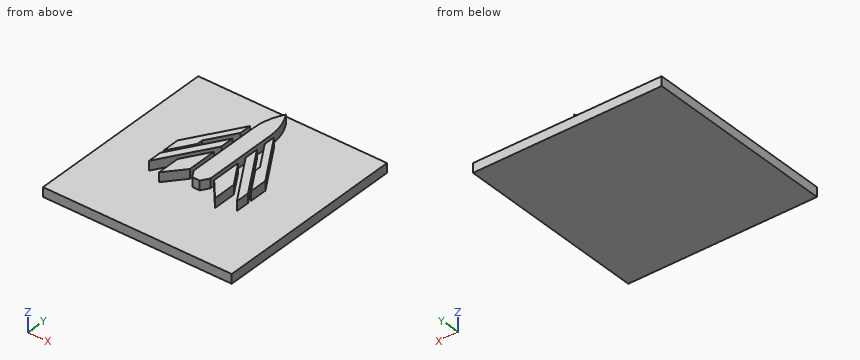
```python
from build123d import *

# Parameters (mm, degrees)
PAD_DEPTH    = 10
SKETCH002_W  = 201.991504
SKETCH002_H  = 207.023942
PAD001_DEPTH = 10
PAD002_DEPTH = 10
PAD003_DEPTH = 10
PAD004_DEPTH = 10


with BuildPart() as part:
    # Sketch → Pad (new body)
    with BuildSketch(Plane.XY):
        with BuildLine():
            Line((-9, 62.657148), (-9, -17.342852))
            Line((-9, -17.342852), (-4, -25.342852))
            Line((-4, -25.342852), (4, -25.342852))
            Line((4, -25.342852), (9, -17.342852))
            Line((9, -17.342852), (9, 62.657148))
            ThreePointArc((9, 62.657148), (6.707183, 79.277918), (0, 94.657148))
            ThreePointArc((0, 94.657148), (-6.707183, 79.277918), (-9, 62.657148))
        make_face()
    extrude(amount=PAD_DEPTH)

    # Sketch002 → Pad001 (join)
    with BuildSketch(Plane.XY):
        Rectangle(SKETCH002_W, SKETCH002_H)
    extrude(amount=-PAD001_DEPTH)

    # Sketch001 → Pad002 (join)
    with BuildSketch(Plane.XY):
        Polygon((13, 14.657148), (13, -17.342852), (30, -37.342852), (30, -12.342852), align=None)
        Polygon((-13, 14.657148), (-13, -17.342852), (-30, -37.342852), (-30, -12.342852), align=None)
    extrude(amount=PAD002_DEPTH)

    # Sketch003 → Pad003 (join)
    with BuildSketch(Plane.XY):
        Polygon((13, 24.657148), (13, 39.657148), (47, -14.342852), (47, -29.342852), align=None)
        Polygon((-13, 39.657148), (-13, 24.657148), (-47, -29.342852), (-47, -14.342852), align=None)
    extrude(amount=PAD003_DEPTH)

    # Sketch004 → Pad004 (join)
    with BuildSketch(Plane.XY):
        Polygon((13, 49.997148), (13, 62.657148), (47, 8.657148), (47, -10.342852), (30.983169, 15.095644), (30.983169, 21.435644), align=None)
        Polygon((-13, 62.657148), (-13, 49.997148), (-30.983169, 21.435644), (-30.983169, 15.095644), (-47, -10.342852), (-47, 8.657148), align=None)
    extrude(amount=PAD004_DEPTH)


solid = part.part
```
Read the model definition and answer for the solid it produces. Units are mm, in the model's axes. Round coordinates to 2 decimals unless told otherwise and drop trailing zeros. Write each loop counter-clockwise with the first axis right and the second up, starting at its lowest first coordinate (ties: lowest second). Pieces come first, ordered by that corner, then holes. Notation, with made-up numbers: M 65,39 L 115,39 A10 cw 115,47 Z; hole C 68,35.5 d6. An arc over 180 degrees is marked long. One line per item, written item: value.
Q1. Straight lines are drawn through the part: line 1 (X direction, y = 24, z = 7.75); line 2 (Z direction, x = 40.5, y = -42); line 3 (Y direction, x = -24.5, z = 6.75). For each, find the intervals that lie inside material, in ascending order. Write a range as [from, to].
Data:
line 1: [-37.34, -29.37], [-22.86, -13.41], [-9, 9], [13.41, 22.86], [29.37, 37.34]
line 2: [-10, 0]
line 3: [-30.87, -3.61], [6.39, 21.39], [31.73, 44.39]
Q2. Find section D-D on x = -53.5. Write down the section's boundary in (y, z).
Data:
outline: M -103.51,-10 L 103.51,-10 L 103.51,0 L -103.51,0 Z
Q3. Find section C-C on x = 37. Write down the section's boundary in (y, z).
Data:
outline: M -103.51,-10 L 103.51,-10 L 103.51,0 L 24.54,0 L 24.54,10 L 5.54,10 L 5.54,0 L 1.54,0 L 1.54,10 L -13.46,10 L -13.46,0 L -103.51,0 Z
Q4. Find section A-A on z = 7. Count the separate pieces of the cut face and the enclosed holes in it, plus the area to 3 significant figures.
Data:
separate pieces: 7
enclosed holes: 0
area: 4,990 mm2
Q5. Flat-ended cylindrical pins translate along their axes: pin 1 Ø12 at (x, y) = (31.5, 59.5) entering from +Z; pin 2 Ø8 at (y, z) = (-5.5, 7) entering from -X; pin 3 Ø3 at (y, z) = (29.5, 2.5) entering from -X. Find the tip coordinate at first contact, or state that the pin passes through.
Data:
pin 1: z = 0
pin 2: x = -47
pin 3: x = -34.82
